The listing builds one solid part. Answer for the finished solid, in the listing's coordinates (mm). A direction names the side the tool comes from. Give positions to 0.01 mm unless a question says otherwise; leave off trailing zeros. Write each loop counter-clockwise with the first axis right and the second up, starting at its lowest first coordinate (ties: lowest second). Pieces come first, ordered by that corner, then holes. Notation, with made-up numbers: M -38.5,79.25 L -8.5,79.25 A27 ccw -8.5,116.25 Z; hole C 31.25,-35 d6. An arc over 180 degrees is marked long. Answer as a JSON object with one key per item and string values.
```python
from build123d import *

# Parameters (mm, degrees)
SKETCH1_W            = 25
SKETCH1_H            = 15
SKETCH1_W_2          = 20
SKETCH1_H_2          = 10
BOSS_EXTRUDE1_DEPTH  = 5
SKETCH2_R            = 0.5
BOSS_EXTRUDE2_DEPTH  = 2
SKETCH5_W            = 2
SKETCH5_H            = 5
BOSS_EXTRUDE3_DEPTH  = 5
SKETCH9_W            = 25
SKETCH9_H            = 3
BOSS_EXTRUDE6_DEPTH  = 2.5458
BOSS_EXTRUDE11_DEPTH = 25
BOSS_EXTRUDE12_DEPTH = 5
SKETCH13_W           = 15.672382287
SKETCH13_H           = 8.611187453
CUT_EXTRUDE2_DEPTH   = 6.3
SKETCH14_W           = 15.973777952
SKETCH14_H           = 8.468711573
CUT_EXTRUDE4_DEPTH   = 6.3
SKETCH17_W           = 5.109908143
SKETCH17_H           = 0.020831831
CUT_EXTRUDE6_DEPTH   = 6.25
CUT_EXTRUDE9_DEPTH   = 2.75


with BuildPart() as part:
    # Sketch1 → Boss-Extrude1 (new body)
    with BuildSketch(Plane.XY):
        with Locations((10.101524963, 5.045869423)):
            Rectangle(SKETCH1_W, SKETCH1_H)
        with Locations((10, 5)):
            Rectangle(SKETCH1_W_2, SKETCH1_H_2, mode=Mode.SUBTRACT)
    extrude(amount=BOSS_EXTRUDE1_DEPTH)

    # Sketch2 → Boss-Extrude2 (add)
    with BuildSketch(Plane.XZ.offset(2.454130577)):
        with Locations(Location((16.351524963, 2.5, 0), (0, 0, 90))):
            Circle(SKETCH2_R)
        with Locations(Location((3.851524963, 2.5, 0), (0, 0, 90))):
            Circle(SKETCH2_R)
    extrude(amount=BOSS_EXTRUDE2_DEPTH)

    # Sketch4 → Revolve1 (revolve)
    with BuildSketch(Plane.ZY.offset(-3.851524963)):
        with BuildLine():
            Line((2.5, -4.454130577), (2.5, -3.954130577))
            ThreePointArc((2.5, -3.954130577), (-0.231202032, -5.265401389), (-0.915920918, -8.216681744))
            Line((-0.915920918, -8.216681744), (-0.431201702, -8.092923646))
            ThreePointArc((-0.431201702, -8.092923646), (0.163723132, -5.572160759), (2.5, -4.454130577))
        make_face()
    revolve1 = revolve(axis=Axis((3.851524963, -4.454130577, 2.5), (0, 1, 0)))

    # Mirror1: Revolve1 across plane
    add(revolve1.mirror(Plane.ZY.offset(-10.101524963)))

    # Sketch5 → Boss-Extrude3 (add)
    with BuildSketch(Plane.XZ.offset(-10)):
        with Locations((10.101524963, 2.5)):
            Rectangle(SKETCH5_W, SKETCH5_H)
    extrude(amount=BOSS_EXTRUDE3_DEPTH)

    # Sketch9 → Boss-Extrude6 (add)
    with BuildSketch(Plane(origin=(0, 12.545869423, 0), x_dir=(1, 0, 0), z_dir=(0, 1, 0))):
        with Locations((10.101524963, 1.5)):
            Rectangle(SKETCH9_W, SKETCH9_H)
    extrude(amount=-BOSS_EXTRUDE6_DEPTH)

    # Sketch10 → Boss-Extrude11 (add)
    with BuildSketch(Plane.ZY.offset(2.398475037)):
        with BuildLine():
            Line((-3, 20.545869423), (-3, 15.545869423))
            ThreePointArc((-3, 15.545869423), (-1.560121709, 14.045869423), (-3, 12.545869423))
            Line((-3, 12.545869423), (2.109908143, 12.545869423))
            Line((2.109908143, 12.545869423), (2.109908143, 14.812382809))
            Line((2.109908143, 14.812382809), (1.14185951, 18.112167841))
            Line((1.14185951, 18.112167841), (-2.398491653, 20.545869423))
            Line((-2.398491653, 20.545869423), (-3, 20.545869423))
        make_face()
    extrude(amount=-BOSS_EXTRUDE11_DEPTH)

    # Sketch11 → Boss-Extrude12 (add)
    with BuildSketch(Plane(origin=(0, 20.545869423, 0), x_dir=(1, 0, 0), z_dir=(0, 1, 0))):
        Polygon((22.601524963, 6.370034263), (22.218498761, 6.583454581), (22.206504106, 6.145147118), (21.839800975, 6.36430085), (21.839800975, 5.944815365), (21.470908859, 6.165277305), (21.470908859, 5.751252067), (21.090285371, 5.978725057), (21.090285371, 5.559686479), (20.715009404, 5.783963617), (20.715009404, 5.37871548), (20.340220839, 5.60270133), (20.340220839, 5.205623066), (19.969772082, 5.427015305), (19.969772082, 5.041871154), (19.609473543, 5.257197293), (19.609473543, 4.889453606), (19.240036756, 5.110241059), (19.204018954, 4.725841041), (18.84343083, 4.941340245), (18.809044063, 4.574347447), (18.482899309, 4.833590643), (18.434301365, 4.437674053), (18.099284993, 4.703969045), (18.029565103, 4.297643206), (17.685889029, 4.570821549), (17.636576293, 4.169081713), (17.36430182, 4.468570031), (17.241504215, 4.047072227), (16.949921416, 4.338518658), (16.830217977, 3.927641452), (16.56189014, 4.222788666), (16.445356586, 3.82279196), (16.205334691, 4.102534079), (16.03541914, 3.718356506), (15.784012514, 4.011367368), (15.609927315, 3.617762258), (15.397544049, 3.917976793), (15.227764955, 3.53410775), (15.005332386, 3.848527484), (14.830770329, 3.453844203), (14.601445444, 3.778006576), (14.424838392, 3.378699578), (14.190795155, 3.709531583), (14.01395843, 3.309705298), (13.77195079, 3.65179539), (13.592594218, 3.246271753), (13.353481935, 3.584269111), (13.179653394, 3.191244304), (12.937387652, 3.533699238), (12.7645906, 3.143006617), (12.501662523, 3.493899949), (12.3122286, 3.098460835), (12.055758175, 3.454101418), (11.859127953, 3.062190893), (11.619872014, 3.416106336), (11.44208312, 3.03616005), (11.201398975, 3.392188142), (11.025924275, 3.017187439), (10.777585982, 3.384537806), (10.557631993, 3.017187439), (10.355137202, 3.367185629), (10.101524963, 3.017187439), (9.847912725, 3.367185629), (9.61814049, 3.017187439), (9.425463944, 3.384537806), (9.177125651, 3.017187439), (9.001650951, 3.392188142), (8.760966807, 3.03616005), (8.583177912, 3.416106336), (8.343921973, 3.062190893), (8.147291751, 3.454101418), (7.890821326, 3.098460835), (7.701387404, 3.493899949), (7.438459327, 3.143006617), (7.265662275, 3.533699238), (7.023396532, 3.191244304), (6.849567992, 3.584269111), (6.610455709, 3.246271753), (6.431099137, 3.65179539), (6.189091497, 3.309705298), (6.012254772, 3.709531583), (5.778211534, 3.378699578), (5.601604482, 3.778006576), (5.372279597, 3.453844203), (5.19771754, 3.848527484), (4.975284972, 3.53410775), (4.805505878, 3.917976793), (4.593122611, 3.617762258), (4.419037412, 4.011367368), (4.167630787, 3.718356506), (3.997715235, 4.102534079), (3.757693341, 3.82279196), (3.641159786, 4.222788666), (3.37283195, 3.927641452), (3.253128511, 4.338518658), (2.961545711, 4.047072227), (2.838748106, 4.468570031), (2.566473633, 4.169081713), (2.517160897, 4.570821549), (2.173484824, 4.297643206), (2.103764933, 4.703969045), (1.768748562, 4.437674053), (1.720150617, 4.833590643), (1.394005864, 4.574347447), (1.359619096, 4.941340245), (0.999030973, 4.725841041), (0.96301317, 5.110241059), (0.593576383, 4.889453606), (0.593576383, 5.257197293), (0.233277844, 5.041871154), (0.233277844, 5.427015305), (-0.137170912, 5.205623066), (-0.137170912, 5.60270133), (-0.511959477, 5.37871548), (-0.511959477, 5.783963617), (-0.887235445, 5.559686479), (-0.887235445, 5.978725057), (-1.267858932, 5.751252067), (-1.267858932, 6.165277305), (-1.636751048, 5.944815365), (-1.636751048, 6.36430085), (-2.00345418, 6.145147118), (-2.015448835, 6.583454581), (-2.398475037, 6.370034263), (-2.398475037, 3), (22.601524963, 3), align=None)
    extrude(amount=-BOSS_EXTRUDE12_DEPTH)

    # Sketch13 → Cut-Extrude2 (cut)
    with BuildSketch(Plane.ZY.offset(2.398475037)):
        with Locations((0.217053265, 16.85146315)):
            Rectangle(SKETCH13_W, SKETCH13_H)
    extrude(amount=-CUT_EXTRUDE2_DEPTH, mode=Mode.SUBTRACT)

    # Sketch14 → Cut-Extrude4 (cut)
    with BuildSketch(Plane(origin=(22.601524963, 0, 0), x_dir=(0, 0, -1), z_dir=(1, 0, 0))):
        with Locations((-0.130094813, 16.801057041)):
            Rectangle(SKETCH14_W, SKETCH14_H)
    extrude(amount=-CUT_EXTRUDE4_DEPTH, mode=Mode.SUBTRACT)

    # Sketch17 → Cut-Extrude6 (cut)
    with BuildSketch(Plane(origin=(22.601524963, 0, 0), x_dir=(0, 0, -1), z_dir=(1, 0, 0))):
        with Locations((0.445045928, 12.556285339)):
            Rectangle(SKETCH17_W, SKETCH17_H)
    extrude(amount=-CUT_EXTRUDE6_DEPTH, mode=Mode.SUBTRACT)

    # Sketch21 → Cut-Extrude9 (cut)
    with BuildSketch(Plane(origin=(0, 12.545869423, 0), x_dir=(1, 0, 0), z_dir=(0, 1, 0))):
        Polygon((-2.398475037, -0.181001123), (-2.398475037, 3), (2.705080675, 3), align=None)
        Polygon((17.294919325, 3), (22.601524963, 3), (22.601524963, 0.170691666), align=None)
    extrude(amount=-CUT_EXTRUDE9_DEPTH, mode=Mode.SUBTRACT)


solid = part.part
```
1. For faces 1 (the flat face through (16.302, 17, -1)), 2 (the flat face through (10, 5, 3)), 3 (the cylindrical face through (4.34, -3.21, 2.39)), 4 (the flat face through (10, 11, -3)), 5 (the flat face through (10, 7, 5)), determine the directions among +Z, -Z, +X, -X, +Y, -Y from which every point of the face is accessible in a straight line to the end or side of a thin tool.
Verdict:
{"face 1": "+Z, -Z, +X, +Y", "face 2": "+Z, -Z", "face 3": "none", "face 4": "-Z, +X, -X, -Y", "face 5": "+Z, +X, -X, +Y"}
2. Consider line 1 along Y through (x, z) = (9, 4); line 2 along X through (y, z) = (1.75, 3); line 3 along Y through (x, z) = (2.5, 0.25). Determine where each line is inside the solid, lowest interval first.
Verdict:
{"line 1": "y = -2.45 to 0, 10 to 12.55", "line 2": "x = -2.4 to 0, 20 to 22.6", "line 3": "y = -6 to -5.14, -2.45 to 0, 10 to 12.55"}
3. A cutting plane is placed at C-C, the plane y = 11.25. Give the vertices of the cut face in (x, z).
Verdict:
{"outline": "M -2.4,0.18 L 2.71,-3 L 17.29,-3 L 22.6,-0.17 L 22.6,5 L -2.4,5 Z"}
4. A cutting plane is placed at D-D, the plane x = -1. Give the vertices of the cut face in (y, z).
Verdict:
{"outline": "M -2.45,0 L 10,0 L 10,-0.69 L 12.55,-0.69 L 12.55,5 L -2.45,5 Z"}
5. A cutting plane is placed at B-B, the plane z = 1.5. Count the separate pieces of the cut face and the enclosed holes in it, plus the area to 3 significant figures.
Verdict:
{"separate pieces": "3", "enclosed holes": "1", "area": "251 mm2"}
6. The mould has two halves that part along X. Classify faces 6 (the flat face through (19.985, 11.291, -1.566)), 7 (the flat face through (10, 20.546, -2.9)), 8 (the flat face through (20, 5, 2)): released by +X, released by -X, zero draft, split by the parting line, or undercut.
Verdict:
{"face 6": "released by +X", "face 7": "zero draft", "face 8": "undercut"}
7. Flat-ended cylindrical pins translate along their axes: pin 1 (3 mm diameter, centred on y = 16.5, z = -1, fed in from +X); pin 2 (2.5 mm diameter, centred on x = 4, z = 1.5, fed in from +Y); pin 3 (12 mm diameter, centred on x = 10.5, y = 8.5, fed in from +Z). Find the tip coordinate at first contact, or state that the pin passes through.
Verdict:
{"pin 1": "stops at x = 16.3", "pin 2": "stops at y = 18.73", "pin 3": "stops at z = 5"}
8. A cutting plane is placed at A-A, the plane y = 6.25. Give the vertices of the cut face in (x, z), plus the area to 3 significant figures.
Verdict:
{"outline": "M -2.4,0 L 0,0 L 0,5 L -2.4,5 Z; M 9.1,0 L 11.1,0 L 11.1,5 L 9.1,5 Z; M 20,0 L 22.6,0 L 22.6,5 L 20,5 Z", "area": "35.0 mm2"}
